Model file for the job. Use its own axes, mm. A direction names the side the tool comes from. Give positions to 0.01 mm unless a question says otherwise; leave off trailing zeros. Use CSV: the item, a comma, the result in double quotes. Start each with the question number.
(1) 3-axis set-ups, long thin cutter, end or side, ignore diameter. For faces 1 (the flat face through (106, -107, 7.938)), 2 (the flat face through (0, -139, 21)), 3 (the cylindrical face through (108.941, -106.572, 2.348)): which of +Z, -Z, +X, -X, +Y, -Y reach the whole face in a straight line?
(2) Drill centre lines: probe 1 along Z at (x, y) = (83, -130); probe 2 along Y at (x, z) = (51, 6.5); probe 3 along Z at (x, y) = (126, -65). Where is each one in solid material? Low to high.
(3) Flat gauge pins, fed straight in: pin 1 (4 mm diameter, centred on x = 104, y = -105.5, fed in from +Z); pin 2 (4 mm diameter, centred on y = -67.5, z = 19, fed in from +X); pin 3 (8 mm diameter, centred on y = -120.5, z = 33, fed in from +X). Where does each tip first touch, or does it go through?
from build123d import *

# Parameters (mm, degrees)
F1_ANGLE = 90


with BuildPart() as f1:
    # F0 (on Front) → F1 (revolve)
    with BuildSketch(Plane.XZ):
        with BuildLine():
            Line((152.4, 4.7625), (152.4, 0))
            Line((152.4, 0), (155.575, 0))
            Line((155.575, 0), (155.575, 7.9375))
            Line((155.575, 7.9375), (148.195857, 7.9375))
            ThreePointArc((148.195857, 7.9375), (137.447355, 27.85258), (122.85325, 45.148614))
            ThreePointArc((122.85325, 45.148614), (120.488449, 45.222947), (120.65, 42.8625))
            ThreePointArc((120.65, 42.8625), (135.414004, 25.188502), (146.05, 4.7625))
            Line((146.05, 4.7625), (152.4, 4.7625))
        make_face()
    revolve(axis=Axis((0, 0, 21.596912), (0, 0, -1)), revolution_arc=F1_ANGLE)


solid = f1.part
Check result:
1,face 1,"+Z, +X, -Y"
1,face 2,"+Z, -Z, -X, +Y, -Y"
1,face 3,"-Z, -X, +Y"
2,probe 1,"0 to 7.94"
2,probe 2,"-146.98 to -136.11"
2,probe 3,"14.3 to 20.96"
3,pin 1,"z = 12.6"
3,pin 2,"x = 127.55"
3,pin 3,"x = 67.87"
